For this review, use the dimensioned drawing (mm, ordinates from the lowest corner) and the shaded views. A direction names the side the tool comes from. Coordinates: 2 decimals unless noted, no trailing zeros. Order: outer loops, then holes, each group sorted by start corner. A loop starts at its lowest first (then second) coordinate and runs counter-clockwise, first axis right, second up. Notation, with made-up numbers: M -29.75,-16.5 L -18.75,-16.5 A19 ccw -18.75,-12.5 Z; hole C 42,29 d2. An arc over 180 degrees is marked long. Use CSV: the item, a comma, the result in double quotes.
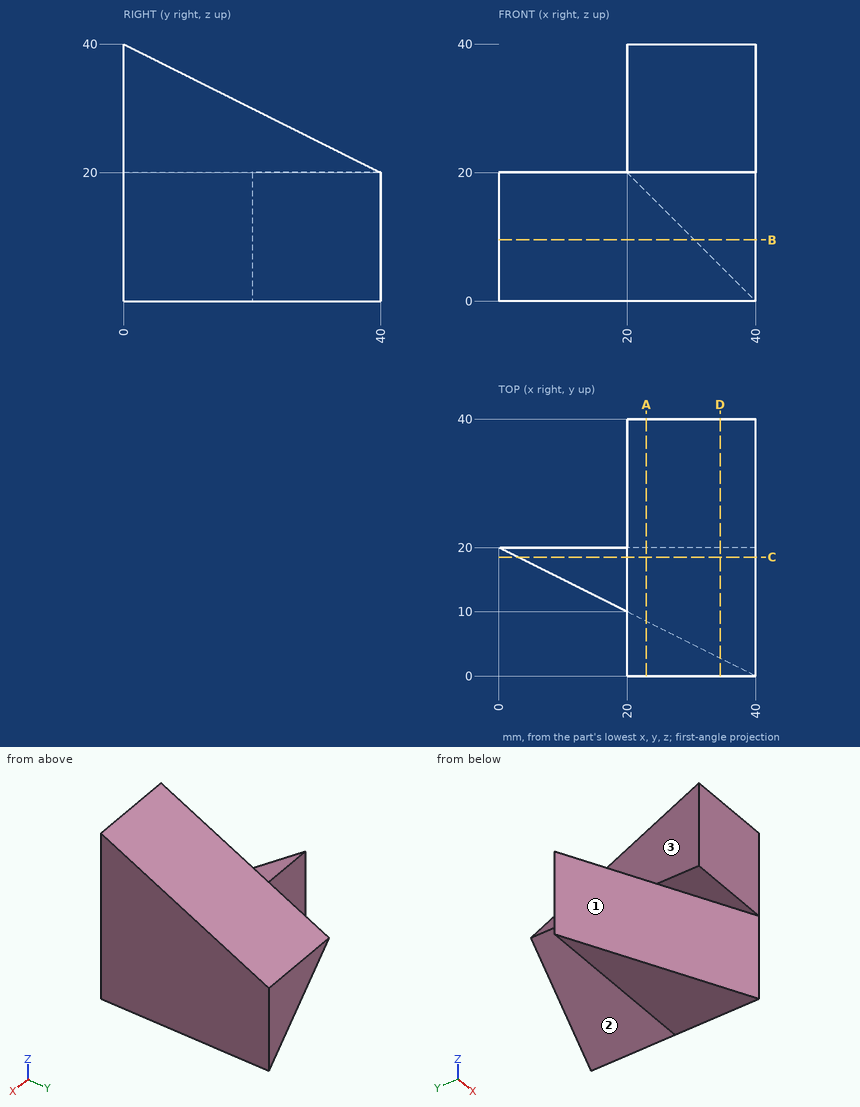
Item 1: Add section C-C on y = 18.5. State the section outline as (x, z) points, and give its area (3 significant figures).
Solutions:
outline,"M 3,0 L 40,0 L 40,30.75 L 20,30.75 L 20,20 L 3,20 Z"
area,"955 mm^2"
Item 2: Clearance check with flat-ended pins moving along their axes: pin 1 Ø10 at (x, y) = (7, 7) entering from +Z; pin 2 Ø11 at (x, y) = (7, 13) entering from +Z; pin 3 Ø8 at (x, z) = (12, 18) entering from -Y. State where each tip first meets the part, or that it passes through.
Solutions:
pin 1,"through"
pin 2,"z = 20"
pin 3,"y = 12"
Item 3: For the marked faces 1, 2 and 3, list the 3-axis set-ups (+Z, -Z, +X, -X, +Y, -Y) from which the entire face can be reached by the end or side of a thin tool; tool diameter is ignored.
Solutions:
face 1,"-Z, -X, -Y"
face 2,"-Z, -X, +Y"
face 3,"+Z, -X, +Y, -Y"
Item 4: Add section A-A on x = 23. State the section outline as (y, z) points.
Solutions:
outline,"M 0,20 L 8.5,20 L 8.5,0 L 20,0 L 20,17 L 40,17 L 40,20 L 0,40 Z"
Item 5: Add section B-B on z = 9.5. State the section outline as (x, y) points.
Solutions:
outline,"M 0,20 L 40,0 L 40,40 L 30.5,40 L 30.5,20 Z"
Item 6: Add section D-D on x = 34.5. State the section outline as (y, z) points, and give its area (4 significant figures).
Solutions:
outline,"M 0,20 L 2.75,20 L 2.75,0 L 20,0 L 20,5.5 L 40,5.5 L 40,20 L 0,40 Z"
area,"1,035 mm^2"
Item 7: To check wall thickness, follow line 1 along X through (y, z) = (32.5, 23); line 2 along Z through (x, y) = (37, 7); line 3 along Y through (x, z) = (37, 30). State the ranges of each line that lie inside material, in increasing order. Write a range as [from, to].
Solutions:
line 1,"[20, 40]"
line 2,"[0, 36.5]"
line 3,"[0, 20]"
